The listing builds one solid part. Answer for the finished solid, in the listing's coordinates (mm). A direction names the side the tool comes from. Coordinates: 2 decimals unless noted, no trailing zeros. Write each loop counter-clockwise with the first axis right and the second up, starting at its lowest first coordinate (ties: lowest second). Pieces come first, ordered by that corner, then holes.
from build123d import *

# Parameters (mm, degrees)
F0_R     = 4.75
F1_DEPTH = 20.55
F4_W     = 9.6
F4_H     = 9.6
F5_DEPTH = 5
F3_W     = 1.5
F3_H     = 10.714468
F6_DEPTH = 5
F7_W     = 6.71751
F7_H     = 6.71751
F8_DEPTH = 5


with BuildPart() as f1:
    # F0 (on Top) → F1 (new body)
    with BuildSketch(Plane.XY):
        Circle(F0_R)
    extrude(amount=F1_DEPTH)

    # F4 (on Top) → F5 (cut)
    with BuildSketch(Plane.XY):
        Rectangle(F4_W, F4_H)
    extrude(amount=F5_DEPTH, mode=Mode.SUBTRACT)

    # F3 (on offset) → F6 (cut)
    with BuildSketch(Plane.XY.offset(20.55)):
        Rectangle(F3_W, F3_H)
    extrude(amount=-F6_DEPTH, mode=Mode.SUBTRACT)

    # F7 (on Top) → F8 (join)
    with BuildSketch(Plane.XY):
        Rectangle(F7_W, F7_H)
    extrude(amount=F8_DEPTH)


solid = f1.part
1. For a pull along X with two mould halves and no side action, classify faces 1 (the flat face through (0.75, 0, 18)), 2 (the flat face through (3.359, 0, 2)), 3 (the flat face through (0, 3.359, 2)) as pulls with the +X half, pulls with the -X half, needs draft (parallel to the pull), parting line crosses it, or undercut.
Results found:
face 1: undercut
face 2: pulls with the +X half
face 3: needs draft
2. Section C-C on x = 0 is taken. Give the vertices of the cut face in (y, z).
Results found:
outline: (-4.75, 5) - (-3.36, 5) - (-3.36, 0) - (3.36, 0) - (3.36, 5) - (4.75, 5) - (4.75, 15.55) - (-4.75, 15.55) - close
3. Find the intervals of material crossed by L1, parallel to Y at x = 1.25, z = 3.5; L2, parallel to Z at x = 0.5, y = 1.5; L3, parallel to X at y = 4.25, z = 19, in increasing order.
Results found:
L1: y = -3.36 to 3.36
L2: z = 0 to 15.55
L3: x = -2.12 to -0.75, 0.75 to 2.12
4. Section D-D on z = 2.25 is taken. Give the vertices of the cut face in (x, y).
Results found:
outline: (-3.36, -3.36) - (3.36, -3.36) - (3.36, 3.36) - (-3.36, 3.36) - close
5. Flat-ended cylindrical pins translate along their axes: P1, Ø1.5, axis at y = 1.5, z = 17.5, coming from the -X side; P2, Ø1, axis at x = -1.5, z = 11.5, coming from the +Y side; P3, Ø1.5, axis at y = -1, z = 17.5, coming from the +X side. Find the tip coordinate at first contact, or state that the pin passes through.
Results found:
P1: stops at x = -4.69
P2: stops at y = 4.64
P3: stops at x = 4.74
6. A tool of negligible diameter and unlimited length cuts with its end or side. For faces 4 (the flat face through (0, -3.359, 2)), 5 (the flat face through (-4, 0, 5)), 6 (the flat face through (-0.75, 0, 18)), from which of +Z, -Z, +X, -X, +Y, -Y can it reach the whole face along a straight path? Write none if from no direction.
Results found:
face 4: -Z, +X, -X, -Y
face 5: -Z, -X, +Y, -Y
face 6: +Z, +Y, -Y
7. Section A-A on y = 0 is taken. Give the vertices of the cut face in (x, z).
Results found:
outline: (-4.75, 5) - (-3.36, 5) - (-3.36, 0) - (3.36, 0) - (3.36, 5) - (4.75, 5) - (4.75, 20.55) - (0.75, 20.55) - (0.75, 15.55) - (-0.75, 15.55) - (-0.75, 20.55) - (-4.75, 20.55) - close
8. Section B-B on z = 18.5 is taken. Give the vertices of the cut face in (x, y).
Results found:
outline: (-0.75, -4.69) - (-0.75, 4.69) arc R4.75 ccw to start; (0.75, -4.69) arc R4.75 ccw to (0.75, 4.69) - close
